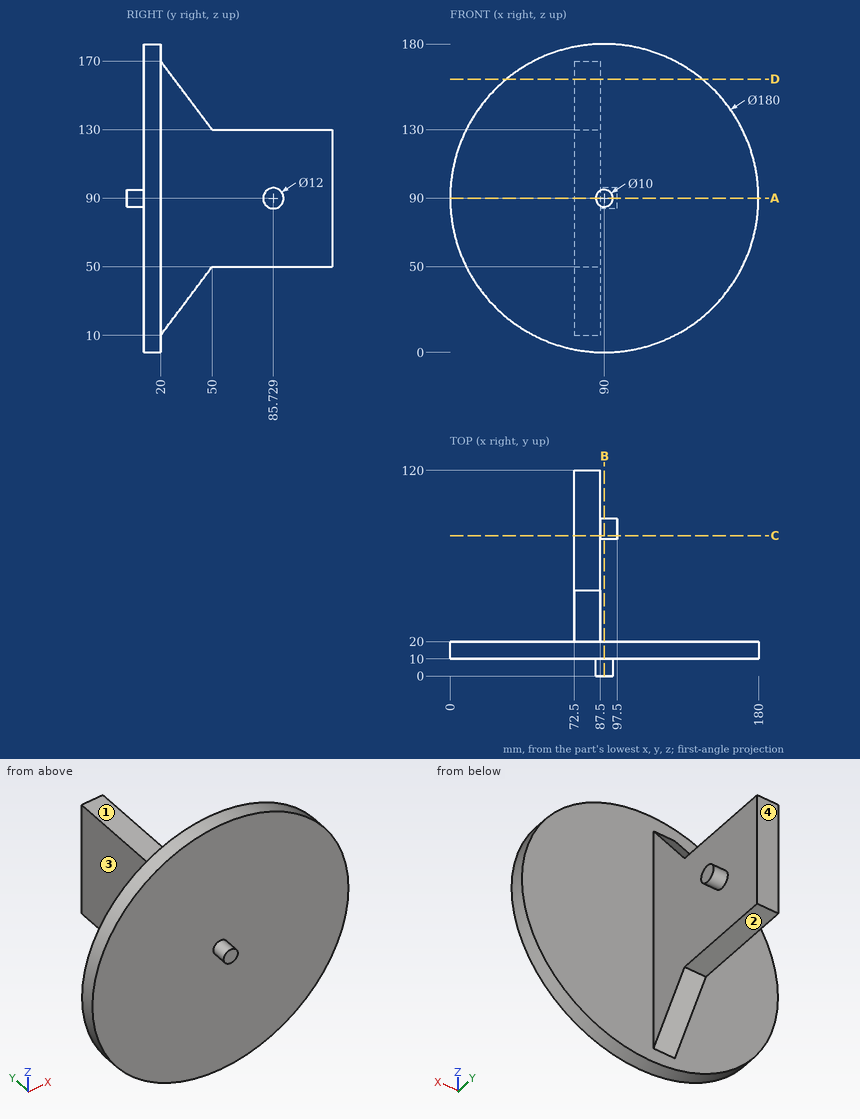
Can you work these out from the drawing? Everything is in mm from the part's minimum corner. A direction names the side the tool comes from. Coordinates: 2 decimals unless noted, no trailing zeros. Write each loop counter-clockwise with the first axis right and the second up, starting at its lowest first coordinate (ties: lowest second). Pieces come first, ordered by that corner, then holes. Notation, with made-up numbers: (-15.75, -30) -> (36.25, -30) arc R24 cw to (36.25, -19) -> close; hole circle Ø5 at (52.5, 48). An arc over 180 degrees is marked (long way). Write item = value, one per line.
(1) Imagine slicing it at D-D (z = 159.5). Please give me the cut outline in (x, y) (3 decimals), and give its area (3 significant figures).
Verdict:
outline = (32.818, 10) -> (147.182, 10) -> (147.182, 20) -> (87.5, 20) -> (87.5, 27.875) -> (72.5, 27.875) -> (72.5, 20) -> (32.818, 20) -> close
area = 1,260 mm^2
(2) If I drill on probe 1 along X at (y, z) = (26.5, 30.5); probe 2 along Y at (x, z) = (113.5, 78.5); probe 3 along Z at (x, y) = (33.5, 15) (1 decimal), over which ranges is the centre line in solid material (lowest first)?
Verdict:
probe_1 = 72.5 to 87.5
probe_2 = 10 to 20
probe_3 = 19.9 to 160.1
(3) On a 3-axis mill with a long thin cutter (end or side, diameter ignored), from which of +Z, -Z, +X, -X, +Y, -Y can I reach the whole of each face in a straight line? I mean the marked faces 1, 2, 3 and 4. Say none if no direction works.
Verdict:
face_1 = +Z, +X, -X, +Y
face_2 = -Z, +X, -X, +Y
face_3 = +Z, -Z, -X, +Y
face_4 = +Z, -Z, +X, -X, +Y
(4) Imagine slicing it at A-A (z = 90). Please give me the cut outline in (x, y), and give its area (3 significant figures).
Verdict:
outline = (0, 10) -> (85, 10) -> (85, 0) -> (95, 0) -> (95, 10) -> (180, 10) -> (180, 20) -> (87.5, 20) -> (87.5, 79.73) -> (97.5, 79.73) -> (97.5, 91.73) -> (87.5, 91.73) -> (87.5, 120) -> (72.5, 120) -> (72.5, 20) -> (0, 20) -> close
area = 3,520 mm^2
(5) Imagine slicing it at C-C (y = 82). Please give me the cut outline in (x, z), and give its area (3 significant figures).
Verdict:
outline = (72.5, 50) -> (87.5, 50) -> (87.5, 85.3) -> (97.5, 85.3) -> (97.5, 94.7) -> (87.5, 94.7) -> (87.5, 130) -> (72.5, 130) -> close
area = 1,290 mm^2
(6) Imagine slicing it at B-B (x = 90). Please give me the cut outline in (y, z), and give its area (3 significant figures).
Verdict:
outline = (0, 85) -> (10, 85) -> (10, 0) -> (20, 0) -> (20, 180) -> (10, 180) -> (10, 95) -> (0, 95) -> close; circle Ø12 at (85.73, 90)
area = 2,010 mm^2
(7) For pin 1 (16.5 mm diameter, centred on x = 77.5, y = 96.5, fed in from -Z); pin 2 (1 mm diameter, centred on y = 89.5, z = 69.5, fed in from +X); pin 3 (5 mm diameter, centred on x = 96.5, z = 143.5, fed in from -Y), each with a flat end and sliding along its axis, tell me the tip position at first contact or that it passes through.
Verdict:
pin_1 = 50
pin_2 = 87.5
pin_3 = 10
